```python
from build123d import *

# Parameters (mm, degrees)
REVOLVE1_ANGLE      = 180
SKETCH2_R           = 24.825
SKETCH2_R_2         = 23
CUT_EXTRUDE1_DEPTH  = 2.15
BOSS_EXTRUDE1_DEPTH = 1.05


with BuildPart() as part:
    # Sketch1 → Revolve1 (revolve)
    with BuildSketch(Plane(origin=(0, 0, 0), x_dir=(1, 0, 0), z_dir=(0, 1, 0))):
        with BuildLine():
            Line((0, 25.25), (0, 23.25))
            ThreePointArc((0, 23.25), (23.25, 0), (0, -23.25))
            Line((0, -23.25), (0, -25.25))
            ThreePointArc((0, -25.25), (25.25, 0), (0, 25.25))
        make_face()
    revolve(axis=Axis((0, 0, 23.25), (0, 0, 1)), revolution_arc=REVOLVE1_ANGLE)

    # Sketch2 → Cut-Extrude1 (cut)
    with BuildSketch(Plane.XZ):
        Circle(SKETCH2_R)
        Circle(SKETCH2_R_2, mode=Mode.SUBTRACT)
    extrude(amount=-CUT_EXTRUDE1_DEPTH, mode=Mode.SUBTRACT)

    # Sketch3 → Boss-Extrude1 (add)
    with BuildSketch(Plane.XZ):
        with BuildLine():
            Line((-5.134436401, 24.288231468), (-5, 23.65228583))
            ThreePointArc((-5, 23.65228583), (0, 24.175), (5, 23.65228583))
            Line((5, 23.65228583), (5, 24.316262562))
            ThreePointArc((5, 24.316262562), (-0.068663834, 24.824905041), (-5.134436401, 24.288231468))
        make_face()
        with BuildLine():
            Line((23.601443665, -7.697563376), (22.983480387, -7.496015896))
            ThreePointArc((22.983480387, -7.496015896), (20.936164136, -12.0875), (17.983480387, -16.156269934))
            Line((17.983480387, -16.156269934), (18.558501104, -16.4882583))
            ThreePointArc((18.558501104, -16.4882583), (21.533330329, -12.352987896), (23.601443665, -7.697563376))
        make_face()
        with BuildLine():
            Line((-18.467007264, -16.590668092), (-17.983480387, -16.156269934))
            ThreePointArc((-17.983480387, -16.156269934), (-20.936164136, -12.0875), (-22.983480387, -7.496015896))
            Line((-22.983480387, -7.496015896), (-23.558501104, -7.828004262))
            ThreePointArc((-23.558501104, -7.828004262), (-21.464666495, -12.471917145), (-18.467007264, -16.590668092))
        make_face()
    extrude(amount=-BOSS_EXTRUDE1_DEPTH)


solid = part.part
```
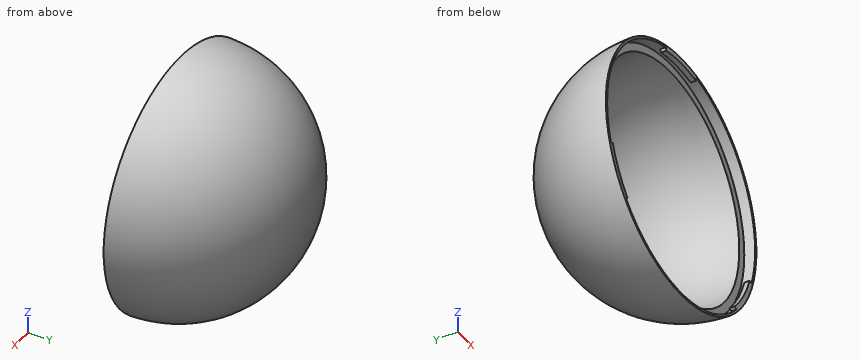
Input: part model. Units: mm. Frame: model coordinates. Give positions to 0.01 mm unless a question says otherwise; leave off trailing zeros. Write each loop counter-clockwise with the first axis right and the second up, starting at its lowest first coordinate (ties: lowest second). Pieces come first, ordered by that corner, then holes. Notation, with made-up numbers: (5, -24) - (53, -24) arc R21 ccw to (53, 9) - close; hole circle Ø5 at (54, 74). An arc over 180 degrees is marked (long way). Write item = value, one per line. Start each with the question number.
1. Section query D-D, the plane y = 22. Output: boundary loops of the cut face in (x, z).
2. Section query C-C, the plane x = -10.5. Output: boundary loops of the cut face in (y, z), then the cut area to 3 significant figures.
3. Section query A-A, the plane z = 0. Output: boundary loops of the cut face in (x, y) (3 decimals), then the cut area to 3 significant figures.
4. Section query B-B, the plane x = 0. Output: boundary loops of the cut face in (y, z) (3 decimals).
5. First-contact query: pin 1 Ø10 at (y, z) = (9.5, 8) entering from +X; pin 2 Ø12 at (x, z) = (-7.5, 2) entering from -Y; pin 3 Ø10 at (x, y) = (11, 18.5) entering from +Z; pin 4 Ø2 at (x, y) = (-14.5, 22.5) entering from -Z. Flat tips, straight axial feed; report the tip coordinate or a pass-through.
6. Ray query, L1, parallel to X at y = 1.35, z = 0 (3 decimals); L2, parallel to X at y = 14.25, z = -0.5; L3, parallel to Z at x = 0, y = 1.6 (3 decimals). Return the intervals inside material, ascending.
Check sheet entries:
q1.outline = circle Ø24.78 at (0, 0); hole circle Ø15.04 at (0, 0)
q2.outline = (0, -22.96) arc R22.96 ccw to (0, 22.96) - (0, 22.5) - (2.15, 22.5) - (2.15, 20.63) arc R20.74 cw to (2.15, -20.63) - (2.15, -22.5) - (0, -22.5) - close
q2.area = 145 mm2
q3.outline = (-25.25, 0) - (-24.825, 0) - (-24.825, 2.15) - (-23.15, 2.15) arc R23.25 cw to (23.15, 2.15) - (24.825, 2.15) - (24.825, 0) - (25.25, 0) arc R25.25 ccw to start
q3.area = 145 mm2
q4.outline = (0, -25.25) arc R25.25 ccw to (0, 25.25) - (0, 24.175) - (1.05, 24.175) - (1.05, 24.825) - (2.15, 24.825) - (2.15, 23.15) arc R23.25 cw to (2.15, -23.15) - (2.15, -24.825) - (0, -24.825) - close
q5.pin_1 = 24.14
q5.pin_2 = 18.74
q5.pin_3 = 19.09
q5.pin_4 = through
q6.L1 = -25.214 to -24.825, 24.825 to 25.214
q6.L2 = -20.84 to -18.36, 18.36 to 20.84
q6.L3 = -25.199 to -24.825, 24.825 to 25.199
